Source: CAD feature listing. Evaluate the final solid. Frame: model axes, mm. Face numbers are marked on the shaded views. A direction names the side the tool comes from. Coordinates: 2 decimals unless noted, no trailing zeros. Loops run counter-clockwise (first coordinate to the right, second up) from the corner with the lowest first, then second, coordinate; pieces in that order, holes last. Notation, with made-up numbers: (63, 12.5) -> (79, 12.5) arc R6 cw to (79, 16.5) -> close; hole circle Ø8 at (-36, 54). An arc over 180 degrees is marked (long way). One line per question, with ' | ' between items. Start each with the question number.
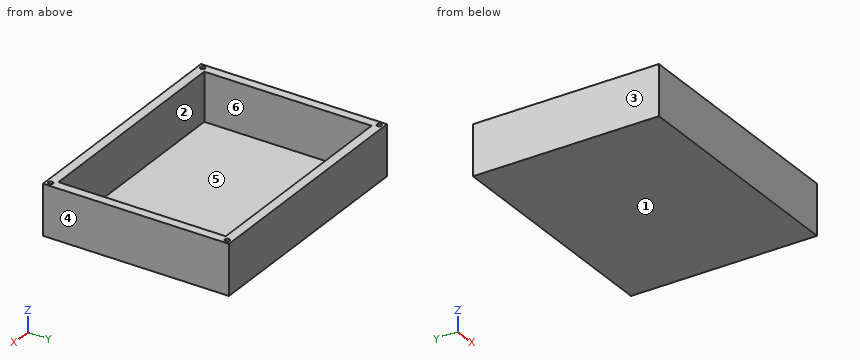
```python
from build123d import *

# Parameters (mm, degrees)
SKETCH_W     = 260
SKETCH_H     = 200
SKETCH_W_2   = 240
SKETCH_H_2   = 180
PAD_DEPTH    = 52
SKETCH001_W  = 260
SKETCH001_H  = 200
PAD001_DEPTH = 2
SKETCH002_R  = 2.5
POCKET_DEPTH = 10


with BuildPart() as part:
    # Sketch → Pad (new body)
    with BuildSketch(Plane.XY):
        with Locations((120.5, 90.5)):
            Rectangle(SKETCH_W, SKETCH_H)
        with Locations((120.5, 90.5)):
            Rectangle(SKETCH_W_2, SKETCH_H_2, mode=Mode.SUBTRACT)
    extrude(amount=PAD_DEPTH)

    # Sketch001 → Pad001 (join)
    with BuildSketch(Plane.XY):
        with Locations((120.5, 90.5)):
            Rectangle(SKETCH001_W, SKETCH001_H)
    extrude(amount=-PAD001_DEPTH)

    # Sketch002 (on Face3 of Pad001) → Pocket (cut)
    with BuildSketch(Plane.XY.offset(52)):
        with Locations((245.5, 185.5)):
            Circle(SKETCH002_R)
        with Locations((245.5, -4.5)):
            Circle(SKETCH002_R)
        with Locations((-4.5, -4.5)):
            Circle(SKETCH002_R)
        with Locations((-4.5, 185.5)):
            Circle(SKETCH002_R)
    extrude(amount=-POCKET_DEPTH, mode=Mode.SUBTRACT)


solid = part.part
```
(1) Contact query for a flat-ended pin moving along its axis: pin 1 Ø1.5 at (x, y) = (244.5, 185.5) entering from +Z. Output: stop coordinate, or through.
(2) Access query for the marked faces 1 and 2. Directions: +Z, -Z, +X, -X, +Y, -Y. A direction counts if a zero-diameter tool reaches every point of the face in a straight line with its end or side. Return the directions, or none.
(3) Draft query along X for the marked faces 3, 4, 5 and 6. Return one class per face: pulls with the +X half, pulls with the -X half, needs draft (parallel to the pull), parting line crosses it, or undercut.
(4) Ray query, L1, parallel to Y at x = 245.5, z = 47.5; L2, parallel to X at y = 185.5, z = 50; L3, parallel to Y at x = -4, z = 49. Return the intervals inside material, ascending.
(5) Cut plane C-C, the plane y = 140. Return the cut outline in (x, z).
(6) Cut plane B-B, the plane x = 21. Return the cut outline in (y, z).
(7) Cut plane A-A, the plane z = 29. Return the cut outline in (x, y).
Here are the results:
1) pin 1: stops at z = 42
2) face 1: -Z, +X, -X, +Y, -Y | face 2: +Z
3) face 3: pulls with the -X half | face 4: pulls with the +X half | face 5: undercut | face 6: undercut
4) L1: y = -9.5 to -7, -2 to 183, 188 to 190.5 | L2: x = -9.5 to -7, -2 to 243, 248 to 250.5 | L3: y = -9.5 to -6.95, -2.05 to 183.05, 187.95 to 190.5
5) outline: (-9.5, -2) -> (250.5, -2) -> (250.5, 52) -> (240.5, 52) -> (240.5, 0) -> (0.5, 0) -> (0.5, 52) -> (-9.5, 52) -> close
6) outline: (-9.5, -2) -> (190.5, -2) -> (190.5, 52) -> (180.5, 52) -> (180.5, 0) -> (0.5, 0) -> (0.5, 52) -> (-9.5, 52) -> close
7) outline: (-9.5, -9.5) -> (250.5, -9.5) -> (250.5, 190.5) -> (-9.5, 190.5) -> close; hole (0.5, 0.5) -> (240.5, 0.5) -> (240.5, 180.5) -> (0.5, 180.5) -> close
